Could you check a few things on this drawing? It's one solid part, dimensions in mm from its lowest x, y, z. A direction names the side the tool comes from. Give positions to 0.01 mm unless a question says otherwise; leave off trailing zeros. Write each loop counter-clockwise with the first axis right and the second up, starting at its lowest first coordinate (ties: lowest second). Pieces come first, ordered by that corner, then holes. Notation, with made-up numbers: M -20,88 L 30,88 A29 cw 30,113 Z; hole C 73.5,-34.75 d1. An arc over 180 degrees is marked long. Write each question's results on one line, items separated by ' | '. Start each with the question number.
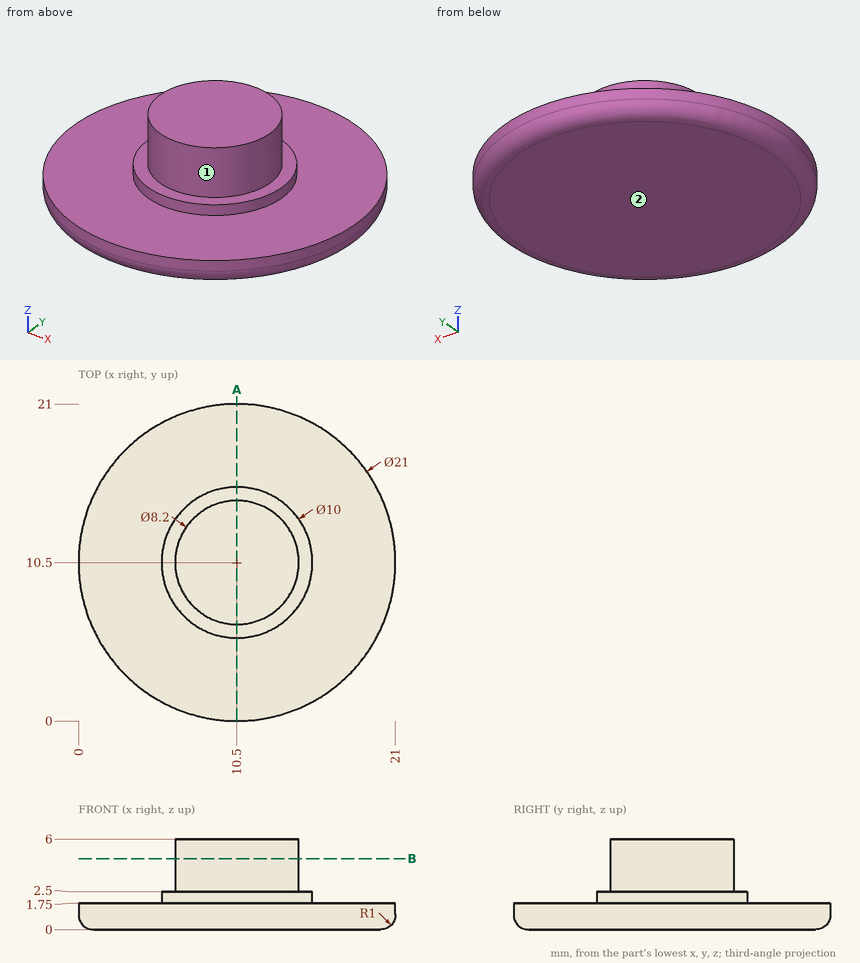
Q1. For the marked faces 1 and 2, which set-ups out of +Z, -Z, +X, -X, +Y, -Y let a thin tool reach every point of the face, with its end or its side?
Q2. If we section it at B-B (z = 4.7): Please give me the cut outline in (x, y), plus the area to 3 significant figures.
Q3. Please list where these lines run through material, in increasing order: line 1 (Z direction, x = 13.5, y = 16); line 2 (X direction, y = 7.5, z = 1.15); line 3 (Y direction, x = 4, z = 0.8). Write a range as [from, to].
Q4. I'm going to push flat-ended pins straight in: P1, Ø3, axis at x = 9, z = 5, coming from the +Y side; P2, Ø1.5, axis at x = 8, z = 5, coming from the -Y side. Where does each tip first touch, or does it pass through?
Q5. If we section it at A-A (x = 10.5): Please give me the cut outline in (y, z).
Determined:
1) face 1: +Z | face 2: -Z, +X, -X, +Y, -Y
2) outline: C 10.5,10.5 d8.2 | area: 52.8 mm²
3) line 1: z = [0, 1.75] | line 2: x = [0.44, 20.56] | line 3: y = [2.28, 18.72]
4) P1: stops at y = 14.6 | P2: stops at y = 6.79
5) outline: M 0,1 A1 ccw 1,0 L 20,0 A1 ccw 21,1 L 21,1.75 L 15.5,1.75 L 15.5,2.5 L 14.6,2.5 L 14.6,6 L 6.4,6 L 6.4,2.5 L 5.5,2.5 L 5.5,1.75 L 0,1.75 Z
